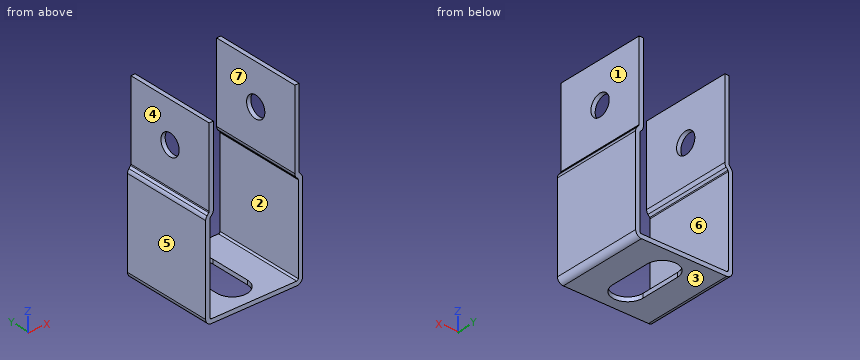
```python
from build123d import *

# Parameters (mm, degrees)
SKETCH1_W                      = 45.72
SKETCH1_H                      = 43.18
BASE_FLANGE1_DEPTH             = 2.0066
EDGE_FLANGE1_STRIP_W           = 9.4996
EDGE_FLANGE1_STRIP_H           = 2.0066
EDGE_FLANGE1_STRIP_CUT_DEPTH   = 43.18
EDGE_FLANGE1_STRIP_2_W         = 9.4996
EDGE_FLANGE1_STRIP_2_H         = 2.0066
EDGE_FLANGE1_STRIP_CUT_2_DEPTH = 43.18
EDGE_FLANGE1_DEPTH             = 43.18
EDGE_FLANGE1_BEND_DEPTH        = 43.18
EDGE_FLANGE2_STRIP_CUT_DEPTH   = 43.18
EDGE_FLANGE2_STRIP_CUT_2_DEPTH = 43.18
EDGE_FLANGE2_DEPTH             = 43.18
EDGE_FLANGE2_BEND_DEPTH        = 43.18
EDGE_FLANGE4_STRIP_CUT_DEPTH   = 43.18
EDGE_FLANGE4_STRIP_CUT_2_DEPTH = 43.18
EDGE_FLANGE4_DEPTH             = 43.18
EDGE_FLANGE4_BEND_DEPTH        = 43.18
F_3_8_CLEARANCE_HOLE3_D        = 10.0838
F_3_8_CLEARANCE_HOLE3_DEPTH    = 25.4
F_3_8_CLEARANCE_HOLE3_TIP      = 3.029479155
F_3_8_CLEARANCE_HOLE4_D        = 10.0838
F_3_8_CLEARANCE_HOLE4_DEPTH    = 25.4
F_3_8_CLEARANCE_HOLE4_TIP      = 3.029479155
CUT_EXTRUDE1_REACH             = 92.157


# Sheet-metal steps are written as plain solids
with BuildPart() as part:
    # Sketch1 → Base-Flange1 (new body)
    with BuildSketch(Plane.XY):
        Rectangle(SKETCH1_W, SKETCH1_H)
    extrude(amount=-BASE_FLANGE1_DEPTH)

    # Edge-Flange1 strip (across the edge) → Edge-Flange1 strip cut (cut)
    with BuildSketch(Plane(origin=(22.86, -21.59, 0), x_dir=(-1, 0, 0), z_dir=(0, 1, 0))):
        with Locations((-2.0066, -1.0033)):
            Rectangle(EDGE_FLANGE1_STRIP_W, EDGE_FLANGE1_STRIP_H)
    extrude(amount=EDGE_FLANGE1_STRIP_CUT_DEPTH, mode=Mode.SUBTRACT)

    # Edge-Flange1 strip 2 (across the edge) → Edge-Flange1 strip cut 2 (cut)
    with BuildSketch(Plane(origin=(-22.86, 21.59, 0), x_dir=(1, 0, 0), z_dir=(0, -1, 0))):
        with Locations((-2.0066, -1.0033)):
            Rectangle(EDGE_FLANGE1_STRIP_2_W, EDGE_FLANGE1_STRIP_2_H)
    extrude(amount=EDGE_FLANGE1_STRIP_CUT_2_DEPTH, mode=Mode.SUBTRACT)

    # Edge-Flange1 section (across the edge) → Edge-Flange1 (add)
    with BuildSketch(Plane(origin=(22.86, -21.59, 0), x_dir=(-1, 0, 0), z_dir=(0, 1, 0))):
        with BuildLine():
            Line((0, 0.7366), (0, 42.4434))
            Line((0, 42.4434), (2.0066, 42.4434))
            Line((2.0066, 42.4434), (2.0066, 0.7366))
            ThreePointArc((2.0066, 0.7366), (2.222345145, 0.215745145), (2.7432, 0))
            Line((2.7432, 0), (2.7432, -2.0066))
            ThreePointArc((2.7432, -2.0066), (0.803464678, -1.203135322), (0, 0.7366))
        make_face()
    extrude(amount=EDGE_FLANGE1_DEPTH)

    # Edge-Flange1 section 2 (across the edge) → Edge-Flange1 bend (add)
    with BuildSketch(Plane(origin=(-22.86, 21.59, 0), x_dir=(1, 0, 0), z_dir=(0, -1, 0))):
        with BuildLine():
            Line((0, 0.7366), (0, 42.4434))
            Line((0, 42.4434), (2.0066, 42.4434))
            Line((2.0066, 42.4434), (2.0066, 0.7366))
            ThreePointArc((2.0066, 0.7366), (2.222345145, 0.215745145), (2.7432, 0))
            Line((2.7432, 0), (2.7432, -2.0066))
            ThreePointArc((2.7432, -2.0066), (0.803464678, -1.203135322), (0, 0.7366))
        make_face()
    extrude(amount=EDGE_FLANGE1_BEND_DEPTH)

    # Edge-Flange2 strip (across the edge) → Edge-Flange2 strip cut (cut)
    with BuildSketch(Plane(origin=(20.8534, -21.59, 42.4434), x_dir=(-0.7660444431189839, 0, -0.6427876096865324), z_dir=(0, 1, 0))):
        Polygon((-7.471038293, 5.781921296), (-1.364813116, -1.495194496), (0.172331663, -0.205376879), (-5.933893514, 7.071738913), align=None)
    extrude(amount=EDGE_FLANGE2_STRIP_CUT_DEPTH, mode=Mode.SUBTRACT)

    # Edge-Flange2 strip 2 (across the edge) → Edge-Flange2 strip cut 2 (cut)
    with BuildSketch(Plane(origin=(-20.8534, 21.59, 42.4434), x_dir=(0.7660444431189839, 0, -0.6427876096865324), z_dir=(0, -1, 0))):
        Polygon((-7.471038293, 5.781921296), (-1.364813116, -1.495194496), (0.172331663, -0.205376879), (-5.933893514, 7.071738913), align=None)
    extrude(amount=EDGE_FLANGE2_STRIP_CUT_2_DEPTH, mode=Mode.SUBTRACT)

    # Edge-Flange2 section (across the edge) → Edge-Flange2 (add)
    with BuildSketch(Plane(origin=(20.8534, -21.59, 42.4434), x_dir=(-0.7660444431189839, 0, -0.6427876096865324), z_dir=(0, 1, 0))):
        with BuildLine():
            Line((-2.0066, 0.268100475), (-2.0066, 1.809657328))
            Line((-2.0066, 1.809657328), (0, 1.809657328))
            Line((0, 1.809657328), (0, 0.268100475))
            ThreePointArc((0, 0.268100475), (0.044422416, 0.016168437), (0.172331663, -0.205376879))
            Line((0.172331663, -0.205376879), (-1.364813116, -1.495194496))
            ThreePointArc((-1.364813116, -1.495194496), (-1.841164797, -0.670129183), (-2.0066, 0.268100475))
        make_face()
    extrude(amount=EDGE_FLANGE2_DEPTH)

    # Edge-Flange2 section 2 (across the edge) → Edge-Flange2 bend (add)
    with BuildSketch(Plane(origin=(-20.8534, 21.59, 42.4434), x_dir=(0.7660444431189839, 0, -0.6427876096865324), z_dir=(0, -1, 0))):
        with BuildLine():
            Line((-2.0066, 0.268100475), (-2.0066, 1.809657328))
            Line((-2.0066, 1.809657328), (0, 1.809657328))
            Line((0, 1.809657328), (0, 0.268100475))
            ThreePointArc((0, 0.268100475), (0.044422416, 0.016168437), (0.172331663, -0.205376879))
            Line((0.172331663, -0.205376879), (-1.364813116, -1.495194496))
            ThreePointArc((-1.364813116, -1.495194496), (-1.841164797, -0.670129183), (-2.0066, 0.268100475))
        make_face()
    extrude(amount=EDGE_FLANGE2_BEND_DEPTH)

    # Edge-Flange4 strip (across the edge) → Edge-Flange4 strip cut (cut)
    with BuildSketch(Plane(origin=(-21.227319471, -21.59, 45.119495558), x_dir=(-1, 0, 0), z_dir=(0, 1, 0))):
        Polygon((-7.471038293, 5.781921296), (-1.364813116, -1.495194496), (0.172331663, -0.205376879), (-5.933893514, 7.071738913), align=None)
    extrude(amount=EDGE_FLANGE4_STRIP_CUT_DEPTH, mode=Mode.SUBTRACT)

    # Edge-Flange4 strip 2 (across the edge) → Edge-Flange4 strip cut 2 (cut)
    with BuildSketch(Plane(origin=(21.227319471, 21.59, 45.119495558), x_dir=(1, 0, 0), z_dir=(0, -1, 0))):
        Polygon((-7.471038293, 5.781921296), (-1.364813116, -1.495194496), (0.172331663, -0.205376879), (-5.933893514, 7.071738913), align=None)
    extrude(amount=EDGE_FLANGE4_STRIP_CUT_2_DEPTH, mode=Mode.SUBTRACT)

    # Edge-Flange4 section (across the edge) → Edge-Flange4 (add)
    with BuildSketch(Plane(origin=(-21.227319471, -21.59, 45.119495558), x_dir=(-1, 0, 0), z_dir=(0, 1, 0))):
        with BuildLine():
            Line((-2.0066, 0.268100475), (-2.0066, 37.369657328))
            Line((-2.0066, 37.369657328), (0, 37.369657328))
            Line((0, 37.369657328), (0, 0.268100475))
            ThreePointArc((0, 0.268100475), (0.044422416, 0.016168437), (0.172331663, -0.205376879))
            Line((0.172331663, -0.205376879), (-1.364813116, -1.495194496))
            ThreePointArc((-1.364813116, -1.495194496), (-1.841164797, -0.670129183), (-2.0066, 0.268100475))
        make_face()
    extrude(amount=EDGE_FLANGE4_DEPTH)

    # Edge-Flange4 section 2 (across the edge) → Edge-Flange4 bend (add)
    with BuildSketch(Plane(origin=(21.227319471, 21.59, 45.119495558), x_dir=(1, 0, 0), z_dir=(0, -1, 0))):
        with BuildLine():
            Line((-2.0066, 0.268100475), (-2.0066, 37.369657328))
            Line((-2.0066, 37.369657328), (0, 37.369657328))
            Line((0, 37.369657328), (0, 0.268100475))
            ThreePointArc((0, 0.268100475), (0.044422416, 0.016168437), (0.172331663, -0.205376879))
            Line((0.172331663, -0.205376879), (-1.364813116, -1.495194496))
            ThreePointArc((-1.364813116, -1.495194496), (-1.841164797, -0.670129183), (-2.0066, 0.268100475))
        make_face()
    extrude(amount=EDGE_FLANGE4_BEND_DEPTH)

    # 3/8 Clearance Hole3
    with Locations(Plane.ZY.offset(21.227319471)):
        with Locations((63.439152886, 0)):
            Hole(F_3_8_CLEARANCE_HOLE3_D / 2, depth=F_3_8_CLEARANCE_HOLE3_DEPTH)
            with Locations((0, 0, -(F_3_8_CLEARANCE_HOLE3_DEPTH + F_3_8_CLEARANCE_HOLE3_TIP / 2))):  # 118° drill point
                Cone(0, F_3_8_CLEARANCE_HOLE3_D / 2, F_3_8_CLEARANCE_HOLE3_TIP, mode=Mode.SUBTRACT)

    # 3/8 Clearance Hole4
    with Locations(Plane(origin=(21.227319471, 0, 0), x_dir=(0, 0, -1), z_dir=(1, 0, 0))):
        with Locations((-63.439152886, 0)):
            Hole(F_3_8_CLEARANCE_HOLE4_D / 2, depth=F_3_8_CLEARANCE_HOLE4_DEPTH)
            with Locations((0, 0, -(F_3_8_CLEARANCE_HOLE4_DEPTH + F_3_8_CLEARANCE_HOLE4_TIP / 2))):  # 118° drill point
                Cone(0, F_3_8_CLEARANCE_HOLE4_D / 2, F_3_8_CLEARANCE_HOLE4_TIP, mode=Mode.SUBTRACT)

    # Sketch38 → Cut-Extrude1 (cut, up to next)
    with BuildSketch(Plane(origin=(0, 0, -2.0066), x_dir=(-1, 0, 0), z_dir=(0, 0, -1)), mode=Mode.PRIVATE) as cut_extrude1_sk1:
        with BuildLine():
            Line((-7.14375, -9.525), (-7.14375, 9.525))
            ThreePointArc((-7.14375, 9.525), (0, 16.66875), (7.14375, 9.525))
            Line((7.14375, 9.525), (7.14375, -9.525))
            ThreePointArc((7.14375, -9.525), (0, -16.66875), (-7.14375, -9.525))
        make_face()
    cut_extrude1_tool1 = extrude(cut_extrude1_sk1.sketch, amount=-CUT_EXTRUDE1_REACH, mode=Mode.PRIVATE) & part.part
    add(cut_extrude1_tool1.solids().sort_by_distance((0, 0, -2.0066))[0], mode=Mode.SUBTRACT)


solid = part.part
```
Input: part model. Units: mm. Frame: model coordinates. Face numbers are marked on the shaded views. A direction names the side the tool comes from. Round coordinates to 2 decimals unless told otherwise and drop trailing zeros. Loops run counter-clockwise (first coordinate to the right, second up) from the corner with the lowest first, then second, coordinate; pieces in that order, holes last.
1) Section query A-A on z = 34.5. Return the cut outline in (x, y), plus the area to 3 significant figures.
Ans:
outline: (-22.86, -21.59) - (-20.85, -21.59) - (-20.85, 21.59) - (-22.86, 21.59) - close; (20.85, -21.59) - (22.86, -21.59) - (22.86, 21.59) - (20.85, 21.59) - close
area: 173 mm2
2) Pin query (flat end, axial travel): pin 1 (12 mm diameter, centred on x = 8.5, y = -10.5, fed in from +Z); pin 2 (11 mm diameter, centred on y = 1, z = 62.5, fed in from -X); pin 3 (2 mm diameter, centred on y = 0.5, z = -1, fed in from +X). Return the tip coordinate at first contact, or that it passes through.
Ans:
pin 1: stops at z = 0
pin 2: stops at x = -21.23
pin 3: stops at x = 22.76
3) Pull-direction query (Z, two-part tool) for the marked faces 1, 2 and 3; classes: released by +Z, released by -Z, zero draft, split by the parting line, or undercut.
Ans:
face 1: zero draft
face 2: undercut
face 3: released by -Z
4) Material intervals for line 1 (X direction, y = 17, z = 76); line 2 (X direction, y = -12, z = 34); line 3 (Z direction, x = 16.5, y = 12), sorted ascending.
Ans:
line 1: x = -21.23 to -19.22, 19.22 to 21.23
line 2: x = -22.86 to -20.85, 20.85 to 22.86
line 3: z = -2.01 to 0
5) Section query D-D on y = -18. Return the cut outline in (x, z).
Ans:
outline: (-22.86, 0.74) arc R2.74 ccw to (-20.12, -2.01) - (20.12, -2.01) arc R2.74 ccw to (22.86, 0.74) - (22.86, 42.18) arc R2.74 ccw to (22.22, 43.94) - (21.4, 44.91) arc R0.74 cw to (21.23, 45.39) - (21.23, 82.49) - (19.22, 82.49) - (19.22, 45.39) arc R2.74 ccw to (19.86, 43.62) - (20.68, 42.65) arc R0.74 cw to (20.85, 42.18) - (20.85, 0.74) arc R0.74 cw to (20.12, 0) - (-20.12, 0) arc R0.74 cw to (-20.85, 0.74) - (-20.85, 42.18) arc R0.74 cw to (-20.68, 42.65) - (-19.86, 43.62) arc R2.74 ccw to (-19.22, 45.39) - (-19.22, 82.49) - (-21.23, 82.49) - (-21.23, 45.39) arc R0.74 cw to (-21.4, 44.91) - (-22.22, 43.94) arc R2.74 ccw to (-22.86, 42.18) - close
6) Set-up query: the marked faces 4, 5, 6 and 7. Return all of +Z, -Z, +X, -X, +Y, -Y with unobstructed straight access to the full face (end or side cutting, diameter ignored); none if empty.
Ans:
face 4: +Z, -X, +Y, -Y
face 5: +Z, -Z, -X, +Y, -Y
face 6: +Y, -Y
face 7: +Z, +Y, -Y
7) Section query B-B on x = 0. Return the cut outline in (y, z), plus the area to 4 significant figures.
Ans:
outline: (-21.59, -2.01) - (-16.67, -2.01) - (-16.67, 0) - (-21.59, 0) - close; (16.67, -2.01) - (21.59, -2.01) - (21.59, 0) - (16.67, 0) - close
area: 19.75 mm2
